from build123d import *

# Parameters (mm, degrees)
F1_DEPTH = 2.5
F3_D     = 4
F4_R     = 10


with BuildPart() as f1:
    # F0 (on Top) → F1 (new body)
    with BuildSketch(Plane.XY):
        with BuildLine():
            ThreePointArc((2.1650635095, -1.25), (2.4148145657, -0.6470476128), (2.5, 0))
            Line((2.5, 0), (0, 0))
            Line((0, 0), (-1.25, -2.1650635095))
            ThreePointArc((-1.25, -2.1650635095), (-0.6470476128, -2.4148145657), (0, -2.5))
            ThreePointArc((0, -2.5), (1.25, -2.1650635095), (2.1650635095, -1.25))
        make_face()
        with BuildLine():
            Line((-1.25, -2.1650635095), (0, 0))
            Line((0, 0), (-1.25, 2.1650635095))
            ThreePointArc((-1.25, 2.1650635095), (-1.767766953, 1.767766953), (-2.1650635095, 1.25))
            ThreePointArc((-2.1650635095, 1.25), (-2.5, 0), (-2.1650635095, -1.25))
            ThreePointArc((-2.1650635095, -1.25), (-1.767766953, -1.767766953), (-1.25, -2.1650635095))
        make_face()
        with BuildLine():
            ThreePointArc((30, -2.5), (31.767766953, -1.767766953), (32.5, 0))
            ThreePointArc((32.5, 0), (31.767766953, 1.767766953), (30, 2.5))
            ThreePointArc((30, 2.5), (28.232233047, 1.767766953), (27.5, 0))
            ThreePointArc((27.5, 0), (28.232233047, -1.767766953), (30, -2.5))
        make_face()
        with BuildLine():
            ThreePointArc((-12.5, 25.9807621135), (-12.5851854343, 26.6278097263), (-12.8349364905, 27.2307621135))
            ThreePointArc((-12.8349364905, 27.2307621135), (-16.25, 28.145825623), (-17.1650635095, 24.7307621135))
            ThreePointArc((-17.1650635095, 24.7307621135), (-15.6470476128, 23.5659475478), (-13.75, 23.8156986041))
            ThreePointArc((-13.75, 23.8156986041), (-12.8349364905, 24.7307621135), (-12.5, 25.9807621135))
        make_face()
        with BuildLine():
            ThreePointArc((-17.1650635095, -24.7307621135), (-16.25, -28.145825623), (-12.8349364905, -27.2307621135))
            ThreePointArc((-12.8349364905, -27.2307621135), (-12.5851854343, -26.6278097263), (-12.5, -25.9807621135))
            ThreePointArc((-12.5, -25.9807621135), (-12.8349364905, -24.7307621135), (-13.75, -23.8156986041))
            ThreePointArc((-13.75, -23.8156986041), (-15.6470476128, -23.5659475478), (-17.1650635095, -24.7307621135))
        make_face()
        with BuildLine():
            ThreePointArc((27.5, 0), (28.232233047, 1.767766953), (30, 2.5))
            Line((30, 2.5), (1.443375673, 2.5))
            Line((1.443375673, 2.5), (2.1650635095, 1.25))
            ThreePointArc((2.1650635095, 1.25), (2.4148145657, 0.6470476128), (2.5, 0))
            Line((2.5, 0), (27.5, 0))
        make_face()
        with BuildLine():
            Line((1.443375673, -2.5), (30, -2.5))
            ThreePointArc((30, -2.5), (28.232233047, -1.767766953), (27.5, 0))
            Line((27.5, 0), (2.5, 0))
            ThreePointArc((2.5, 0), (2.4148145657, -0.6470476128), (2.1650635095, -1.25))
            Line((2.1650635095, -1.25), (1.443375673, -2.5))
        make_face()
        with BuildLine():
            Line((-12.8349364905, -27.2307621135), (1.443375673, -2.5))
            Line((1.443375673, -2.5), (0, -2.5))
            ThreePointArc((0, -2.5), (-0.6470476128, -2.4148145657), (-1.25, -2.1650635095))
            Line((-1.25, -2.1650635095), (-13.75, -23.8156986041))
            ThreePointArc((-13.75, -23.8156986041), (-12.8349364905, -24.7307621135), (-12.5, -25.9807621135))
            ThreePointArc((-12.5, -25.9807621135), (-12.5851854343, -26.6278097263), (-12.8349364905, -27.2307621135))
        make_face()
        with BuildLine():
            Line((0, 2.5), (1.443375673, 2.5))
            Line((1.443375673, 2.5), (-12.8349364905, 27.2307621135))
            ThreePointArc((-12.8349364905, 27.2307621135), (-12.5851854343, 26.6278097263), (-12.5, 25.9807621135))
            ThreePointArc((-12.5, 25.9807621135), (-12.8349364905, 24.7307621135), (-13.75, 23.8156986041))
            Line((-13.75, 23.8156986041), (-1.25, 2.1650635095))
            ThreePointArc((-1.25, 2.1650635095), (-0.6470476128, 2.4148145657), (0, 2.5))
        make_face()
        with BuildLine():
            Line((-13.75, -23.8156986041), (-1.25, -2.1650635095))
            ThreePointArc((-1.25, -2.1650635095), (-1.767766953, -1.767766953), (-2.1650635095, -1.25))
            Line((-2.1650635095, -1.25), (-2.8867513459, 0))
            Line((-2.8867513459, 0), (-17.1650635095, -24.7307621135))
            ThreePointArc((-17.1650635095, -24.7307621135), (-15.6470476128, -23.5659475478), (-13.75, -23.8156986041))
        make_face()
        with BuildLine():
            ThreePointArc((-2.1650635095, 1.25), (-1.767766953, 1.767766953), (-1.25, 2.1650635095))
            Line((-1.25, 2.1650635095), (-13.75, 23.8156986041))
            ThreePointArc((-13.75, 23.8156986041), (-15.6470476128, 23.5659475478), (-17.1650635095, 24.7307621135))
            Line((-17.1650635095, 24.7307621135), (-2.8867513459, 0))
            Line((-2.8867513459, 0), (-2.1650635095, 1.25))
        make_face()
        with BuildLine():
            Line((0, 0), (2.5, 0))
            ThreePointArc((2.5, 0), (2.4148145657, 0.6470476128), (2.1650635095, 1.25))
            ThreePointArc((2.1650635095, 1.25), (1.25, 2.1650635095), (0, 2.5))
            ThreePointArc((0, 2.5), (-0.6470476128, 2.4148145657), (-1.25, 2.1650635095))
            Line((-1.25, 2.1650635095), (0, 0))
        make_face()
        with BuildLine():
            Line((0, -2.5), (1.443375673, -2.5))
            Line((1.443375673, -2.5), (2.1650635095, -1.25))
            ThreePointArc((2.1650635095, -1.25), (1.25, -2.1650635095), (0, -2.5))
        make_face()
        with BuildLine():
            Line((2.1650635095, 1.25), (1.443375673, 2.5))
            Line((1.443375673, 2.5), (0, 2.5))
            ThreePointArc((0, 2.5), (1.25, 2.1650635095), (2.1650635095, 1.25))
        make_face()
        with BuildLine():
            ThreePointArc((-2.1650635095, -1.25), (-2.5, 0), (-2.1650635095, 1.25))
            Line((-2.1650635095, 1.25), (-2.8867513459, 0))
            Line((-2.8867513459, 0), (-2.1650635095, -1.25))
        make_face()
    extrude(amount=F1_DEPTH)

    # F3 (through all)
    with Locations(Plane(origin=(0, 0, 0), x_dir=(1, 0, 0), z_dir=(0, 0, -1))):
        with Locations((0, 0)):
            Hole(F3_D / 2)

    # F4
    f4_edges = [f1.edges().sort_by_distance(p)[0] for p in [
        (1.443376, -2.5, 1.25),
        (-2.886751, 0, 1.25),
        (1.443376, 2.5, 1.25),
    ]]
    fillet(f4_edges, radius=F4_R)


solid = f1.part
Read the model definition and answer for the solid it produces. Units are mm, in the model's axes. A direction names the side the tool comes from. Give positions to 0.01 mm unless a question says otherwise; leave off trailing zeros. Loops run counter-clockwise (first coordinate to the right, second up) from the corner with the lowest first, then second, coordinate; pieces in that order, holes last. Notation, with made-up numbers: (75, 58) -> (93, 58) arc R21 ccw to (93, 66) -> close; hole circle Ø1 at (-19, 89.5). An arc over 180 degrees is marked (long way). Use a Markdown table: item, result.
Q1. Section C-C, the plane x = -7 is taken. Determine the outline of the cut face in (y, z), then the cut area to 3 significant figures.
Solved:
| item | result |
|---|---|
| outline | (-17.12, 0) -> (-7.12, 0) -> (-7.12, 2.5) -> (-17.12, 2.5) -> close; (7.12, 0) -> (17.12, 0) -> (17.12, 2.5) -> (7.12, 2.5) -> close |
| area | 50.0 mm^2 |
Q2. A tool of negligible diameter and unlimited length cuts with its end or side. For faces 1 (the face through (19, 2.5, 1)), 2 (the face through (-11.39, -14.73, 1.23)), 3 (the face through (18, -2.5, 1)), from which of +Z, -Z, +X, -X, +Y, -Y can it reach the whole face along a straight path? Write none if from no direction.
Solved:
| item | result |
|---|---|
| face 1 | +Z, -Z, +X, +Y |
| face 2 | +Z, -Z, -X |
| face 3 | +Z, -Z, +X, -Y |
Q3. Find the intervals of material crossed by line 1 along Y through (x, z) = (-14.5, 1.35); line 2 along Y through (x, z) = (0, 1.95); line 3 along Y through (x, z) = (19.5, 0.4), in increasing order.
Solved:
| item | result |
|---|---|
| line 1 | y = -28.43 to -20.11, 20.11 to 28.43 |
| line 2 | y = -5.58 to -2, 2 to 5.58 |
| line 3 | y = -2.5 to 2.5 |
Q4. Determine the mould class of faces 4 (the face through (-7.219, -17.503, 1.232)), 5 (the face through (-11.549, 15.003, 1.232)), 6 (the face through (2, -2, 0)), 7 (the face through (2.15, 3.88, 1.27)) for opening direction Y: pulls with the +Y half, pulls with the -Y half, needs draft (parallel to the pull), parting line crosses it, or undercut.
Solved:
| item | result |
|---|---|
| face 4 | pulls with the -Y half |
| face 5 | undercut |
| face 6 | needs draft |
| face 7 | pulls with the +Y half |
Q5. Each of these flat-tipped pins is pushed along its axis until it touches: pin 1 (1.2 mm diameter, centred on x = 13.5, z = 2, fed in from -Y); pin 2 (1 mm diameter, centred on x = 23.5, z = 1, fed in from +Y); pin 3 (6.5 mm diameter, centred on x = 0, y = 0, fed in from -Z). Where does it stop, or does it pass through?
Solved:
| item | result |
|---|---|
| pin 1 | stops at y = -2.5 |
| pin 2 | stops at y = 2.5 |
| pin 3 | stops at z = 0 |
Q6. Section B-B, the plane x = -15 is taken. Determine the outline of the cut face in (y, z).
Solved:
| item | result |
|---|---|
| outline | (-28.48, 0) -> (-20.98, 0) -> (-20.98, 2.5) -> (-28.48, 2.5) -> close; (20.98, 0) -> (28.48, 0) -> (28.48, 2.5) -> (20.98, 2.5) -> close |
Q7. Section A-A, the plane z = 0.7 is taken. Determine the outline of the cut face in (x, y), then the cut area to 3 significant figures.
Solved:
| item | result |
|---|---|
| outline | (-17.17, -24.73) arc R2.5 ccw to (-12.83, -27.23) -> (-1.44, -7.5) arc R10 cw to (7.22, -2.5) -> (30, -2.5) arc R2.5 ccw to (30, 2.5) -> (7.22, 2.5) arc R10 cw to (-1.44, 7.5) -> (-12.83, 27.23) arc R2.5 ccw to (-17.17, 24.73) -> (-5.77, 5) arc R10 cw to (-5.77, -5) -> close; hole circle Ø4 at (0, 0) |
| area | 472 mm^2 |
Q8. Section D-D, the plane y = 8.5 is taken. Determine the outline of the cut face in (x, z).
Solved:
| item | result |
|---|---|
| outline | (-7.79, 0) -> (-2.02, 0) -> (-2.02, 2.5) -> (-7.79, 2.5) -> close |
